Autodesk Inventor part; units mm, degrees
ref_plane "YZ Plane" through (0, 0, 0) normal (1, 0, 0) x (0, 1, 0)
ref_plane "XZ Plane" through (0, 0, 0) normal (0, 1, 0) x (-1, 0, 0)
ref_plane "XY Plane" through (0, 0, 0) normal (0, 0, 1) x (1, 0, 0)
ref_plane "Arbeitsebene1" through (0, 0, 0) normal (0, 0, 1) x (1, 0, 0)
sketch "Skizze1" plane through (0, 0, 0) normal (0, 0, 1) x (1, 0, 0)
  circle A0 centre (-44.65, -14) radius 1.4
  circle A1 centre (-44.65, 14) radius 1.4
  circle A2 centre (-8.65, -14) radius 1.4
  circle A3 centre (-8.65, 14) radius 1.4
  circle A4 centre (23.0201, 18.1) radius 1.8
  circle A5 centre (-4.9799, 18.1) radius 1.8
  circle A6 centre (-4.9799, 4) radius 1.8
  circle A7 centre (-4.9799, -4) radius 1.8
  circle A8 centre (-4.9799, -18.1) radius 1.8
  circle A9 centre (23.0201, -18.1) radius 1.8
  circle A10 centre (23.0201, 4) radius 1.8
  circle A11 centre (23.0201, -4) radius 1.8
  circle A12 centre (40.1702, -4) radius 1.8
  circle A13 centre (40.1702, -20.3) radius 1.8
  circle A14 centre (40.1702, 4) radius 1.8
  circle A15 centre (40.1702, 20.3) radius 1.8
  line L0 (-45.5, -24.3) -> (-47.5, -22.3)
  line L1 (40.5, -24.3) -> (-45.5, -24.3)
  line L2 (42.5, -22.3) -> (40.5, -24.3)
  line L3 (42.5, 22.3) -> (42.5, -22.3)
  line L4 (40.5, 24.3) -> (42.5, 22.3)
  line L5 (-45.5, 24.3) -> (40.5, 24.3)
  line L6 (-47.5, 22.3) -> (-45.5, 24.3)
  line L7 (-47.5, -22.3) -> (-47.5, 22.3)
  circle A16 centre (-26.65, 0) radius 10
  point P0 (0, 0)
extrude "Extrusion1" add sketch "Skizze1" along normal blind 1
properties part number "60_Planktoscope_Sampleholder_spacer"
For this review, take the finished solid that the model builds, in its own axes (mm). Round coordinates to 2 decimals unless told otherwise and drop trailing zeros. Write each loop counter-clockwise with the first axis right and the second up, starting at its lowest first coordinate (ties: lowest second). Pieces come first, ordered by that corner, then holes. Notation, with made-up numbers: (0, -33.5) -> (29, -33.5) arc R24 cw to (29, -5.5) -> close; hole circle Ø3 at (71.5, -8.75). An arc over 180 degrees is marked (long way). Use one line per item in the form item = value.
Q1. Consider section B-B (x = -44.65). State the section outline as (y, z) points, then the cut area to 3 significant figures.
Resolved:
outline = (-24.3, 0) -> (-15.4, 0) -> (-15.4, 1) -> (-24.3, 1) -> close; (-12.6, 0) -> (12.6, 0) -> (12.6, 1) -> (-12.6, 1) -> close; (15.4, 0) -> (24.3, 0) -> (24.3, 1) -> (15.4, 1) -> close
area = 43.0 mm²
Q2. To check wall thickness, follow probe 1 along Y at (x, z) = (-44.65, 0.4); probe 2 along X at (y, z) = (-5, 0.1); probe 3 along X at (y, z) = (19, 0.5). State the ranges of each line that lie inside material, in increasing order. Write a range as from..to.
Resolved:
probe_1 = -24.3..-15.4, -12.6..12.6, 15.4..24.3
probe_2 = -47.5..-35.31, -17.99..-6.48, -3.48..21.52, 24.52..38.67, 41.67..42.5
probe_3 = -47.5..-6.54, -3.42..21.46, 24.58..38.93, 41.42..42.5
Q3. Clearance check with a flat-ended pin moving along its axis: pin 1 Ø3 at (x, y) = (-4.98, -4) entering from -Z. State where the tip first meets the part, or that it passes through.
Resolved:
pin_1 = through
Q4. Consider section C-C (z = 0.75). State how many separate pieces and enclosed holes the cut face has, then the cut area to 3 significant figures.
Resolved:
separate_pieces = 1
enclosed_holes = 17
area = 3,910 mm²
Q5. Consider section D-D (x = -26.65). State the section outline as (y, z) points, then the cut area to 3 significant figures.
Resolved:
outline = (-24.3, 0) -> (-10, 0) -> (-10, 1) -> (-24.3, 1) -> close; (10, 0) -> (24.3, 0) -> (24.3, 1) -> (10, 1) -> close
area = 28.6 mm²
Q6. The part is to be moulded in two halves that separate along X. For faces 1 (the cylindrical face through (-43.315, -14.421, 0.493)), 2 (the flat face through (41.5, 23.3, 0.5)), 3 (the flat face through (-46.5, 23.3, 0.5)), say which applies: released by +X, released by -X, zero draft, split by the parting line, or undercut.
Resolved:
face_1 = undercut
face_2 = released by +X
face_3 = released by -X
Q7. Consider section A-A (y = 0). State the section outline as (x, z) points, then the cut area to 3 significant figures.
Resolved:
outline = (-47.5, 0) -> (-36.65, 0) -> (-36.65, 1) -> (-47.5, 1) -> close; (-16.65, 0) -> (42.5, 0) -> (42.5, 1) -> (-16.65, 1) -> close
area = 70.0 mm²
